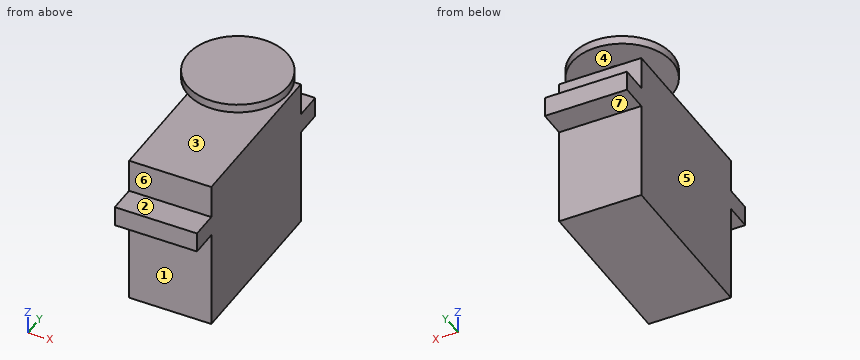
Autodesk Inventor part; units mm, degrees
ref_plane "YZ Plane" through (0, 0, 0) normal (1, 0, 0) x (0, 1, 0)
ref_plane "XZ Plane" through (0, 0, 0) normal (0, 1, 0) x (-1, 0, 0)
ref_plane "XY Plane" through (0, 0, 0) normal (0, 0, 1) x (1, 0, 0)
sketch "Sketch1" plane through (0, 0, 0) normal (0, 0, 1) x (1, 0, 0)
  line L0 (-9.779, -20.1676) -> (9.779, -20.1676)
  line L1 (9.779, -20.1676) -> (9.779, 20.1676)
  line L2 (9.779, 20.1676) -> (-9.779, 20.1676)
  line L3 (-9.779, 20.1676) -> (-9.779, -20.1676)
  line L4 (-9.779, -20.1676) -> (9.779, 20.1676) construction
  line L5 (9.779, -20.1676) -> (-9.779, 20.1676) construction
  point P0 (0, 0)
  dimension "ServoWidth" = 19.558
  dimension "ServoHeight" = 40.3352
extrude "Body" add sketch "Sketch1" along normal mid plane 36.2077
sketch "Sketch2" plane through (0, 0, 18.1038) normal (0, 0, 1) x (1, 0, 0)
  circle A0 centre (0, 10.2616) radius 4.4259
  line L0 (9.779, 20.1676) -> (-9.779, 20.1676)
  point P0 (0, 0)
  dimension "d4" = 8.8519
  dimension "d7" = 9.906
extrude "Actuator" add sketch "Sketch2" along normal blind 4.8514
sketch "Sketch3" plane through (0, 10.2616, 22.9552) normal (0, 0, 1) x (1, 0, 0)
  circle A0 centre (0, 0) radius 11.9444
  point P0 (0, -10.2616)
  dimension "ServoWheelDiameter" = 23.8887
extrude "Wheel" add sketch "Sketch3" along normal blind 2.0193
sketch "Sketch4" plane through (-9.779, -20.1676, 18.1038) normal (-1, 0, 0) x (0, 0, 1)
  line L0 (-7.9375, -6.4389) -> (-12.7, -6.4389)
  line L1 (-12.7, -6.4389) -> (-12.7, 0)
  line L2 (-12.7, 0) -> (-7.9375, 0)
  line L3 (-7.9375, 0) -> (-7.9375, -6.4389)
  line L4 (-7.9375, -6.4389) -> (-12.7, 0) construction
  line L5 (-12.7, -6.4389) -> (-7.9375, 0) construction
  line L6 (-36.2077, 0) -> (0, 0)
  line L7 (0, 40.3352) -> (0, 0)
  line L8 (-12.7, 46.7741) -> (-7.9375, 46.7741)
  line L9 (-7.9375, 46.7741) -> (-7.9375, 40.3352)
  line L10 (-7.9375, 40.3352) -> (-12.7, 40.3352)
  line L11 (-12.7, 40.3352) -> (-12.7, 46.7741)
  line L12 (-12.7, 46.7741) -> (-7.9375, 40.3352) construction
  line L13 (-7.9375, 46.7741) -> (-12.7, 40.3352) construction
  line L14 (-36.2077, 40.3352) -> (0, 40.3352)
  point P0 (-18.1038, 20.1676)
  point P1 (-10.3188, -3.2195)
  point P2 (-10.3188, 43.5546)
  point P3 (-7.9375, 43.5546)
  point P4 (-7.9375, -3.2194)
  dimension "ServoTabWidth" = 4.7625
  dimension "ServoTabHeight" = 6.4389
  dimension "ServoTabDepthOffset" = 7.9375
  dimension "d16" = 6.4389
  dimension "d17" = 4.7625
extrude "Tabs" add sketch "Sketch4" against normal up to surface (19.558 mm away)
equation "\"d16\" = ServoTabHeight"
equation "\"d17\" = ServoTabWidth"
properties part number "Servo"
Design review of the part built by this model. Coordinates are the model's own, in mm. Face numbers are marked on the shaded views. A direction names the side the tool comes from. Give positions to 0.01 mm unless a question says otherwise; leave off trailing zeros. Write each loop counter-clockwise with the first axis right and the second up, starting at its lowest first coordinate (ties: lowest second). Pieces come first, ordered by that corner, then holes. Notation, with made-up numbers: M -18,-5.75 L 14,-5.75 A31 cw 14,19.25 Z; hole C 53,1 d10. An arc over 180 degrees is marked long. Answer as a JSON object with one key per item and string values. Group by question number.
1) We need section D-D (y = -17.5). Give the boundary of the cut face in (x, z).
2) We need section A-A (x = 7.25). Give the boundary of the cut face in (y, z).
3) For line 1 along Z through (x, y) = (3.5, 4.5); line 2 along X through (y, z) = (-8.5, -4.5); line 3 along Z through (x, y) = (2.25, 24.5), list the stretches that pass through material, from the lowest coordinate up.
4) Clearance check with flat-ended pins moving along their axes: pin 1 Ø12 at (y, z) = (-8.5, -0.5) entering from -X; pin 2 Ø5 at (x, y) = (-1.5, 22) entering from -Z; pin 3 Ø10 at (x, z) = (2, -9) entering from -Y; pin 4 Ø10 at (y, z) = (-19, 12) entering from +X. State where each tip first meets the part, or that it passes through.
5) We need section B-B (x = 0). Give the boundary of the cut face in (y, z), and give its area (3 significant figures).
6) Mouldability with a two-part tool opening along Z and no side actions: class the marked faces 1, 2 and 3 as released by +Z, released by -Z, zero draft, split by the parting line, or undercut.
7) We need section C-C (z = -5.5). Give the boundary of the cut face in (x, y), and give its area (3 significant figures).
8) Tool access review of the marked faces 4, 5, 6 and 7: name each direction out of +Z, -Z, +X, -X, +Y, -Y from which nothing blocks a thin tool from reaching the whole face with its end or side.
Answer key:
{
 "1": {"outline": "M -9.78,-18.1 L 9.78,-18.1 L 9.78,18.1 L -9.78,18.1 Z"},
 "2": {"outline": "M -26.61,5.4 L -20.17,5.4 L -20.17,-18.1 L 20.17,-18.1 L 20.17,5.4 L 26.61,5.4 L 26.61,10.17 L 20.17,10.17 L 20.17,18.1 L -20.17,18.1 L -20.17,10.17 L -26.61,10.17 Z; M 0.77,22.96 L 19.75,22.96 L 19.75,24.97 L 0.77,24.97 Z"},
 "3": {"line 1": "z = -18.1 to 18.1, 22.96 to 24.97", "line 2": "x = -9.78 to 9.78", "line 3": "z = 5.4 to 10.17"},
 "4": {"pin 1": "stops at x = -9.78", "pin 2": "stops at z = -18.1", "pin 3": "stops at y = -20.17", "pin 4": "stops at x = 9.78"},
 "5": {"outline": "M -26.61,5.4 L -20.17,5.4 L -20.17,-18.1 L 20.17,-18.1 L 20.17,5.4 L 26.61,5.4 L 26.61,10.17 L 20.17,10.17 L 20.17,18.1 L 14.69,18.1 L 14.69,22.96 L 22.21,22.96 L 22.21,24.97 L -1.68,24.97 L -1.68,22.96 L 5.84,22.96 L 5.84,18.1 L -20.17,18.1 L -20.17,10.17 L -26.61,10.17 Z", "area": "1,610 mm²"},
 "6": {"face 1": "zero draft", "face 2": "released by +Z", "face 3": "undercut"},
 "7": {"outline": "M -9.78,-20.17 L 9.78,-20.17 L 9.78,20.17 L -9.78,20.17 Z", "area": "789 mm²"},
 "8": {"face 4": "none", "face 5": "-Z, -X, +Y, -Y", "face 6": "+Z, +X, -X, -Y", "face 7": "-Z, +X, -X, +Y"}
}
